The model under review builds one solid part; all positions refer to its coordinate system, in mm. Face numbers are marked on the shaded views. Coordinates: 2 decimals unless noted, no trailing zeros. Order: outer loops, then holes, each group sorted by start corner. A loop starts at its lowest first (then second) coordinate and runs counter-clockwise, first axis right, second up. Notation, with made-up numbers: M -6,50.5 L 10,50.5 A17 cw 10,54.5 Z; hole C 9.25,1.5 d11. An arc over 180 degrees is marked long. Answer as CSV lines item,"result". Start each with the question number.
Q1. For P1, Ø1.3, axis at y = 8.5, z = -5, coming from the +X side; P2, Ø2.5, axis at x = 3, y = -0.5, coming from the -Z side; P3, Ø3, axis at x = 24, y = 9.5, coming from the +Z side; P4, Ø1.3, axis at y = -12, z = 1, coming from the -X side, all flat-tipped, find the tip position at first contact; note any pin that passes through.
Q2. Consider section C-C on x = 32. Write out the cut boundary in (y, z), and give its area (3 significant figures).
Q3. Consider section D-D on x = 18.5. Write out the cut boundary in (y, z), and give its area (3 significant figures).
Q4. Wall thickness on L1, parallel to Z at x = 8.6, y = 0; L2, parallel to Y at x = 10.65, z = 0: over which ranges is each line inside the solid? List them lowest first. Write a range as [from, to].
Q5. The part is to be moulded in two halves that separate along Z. For the marked faces 1, 2 and 3, say which applies: +Z half, -Z half, draft (parallel to the pull), parting line (faces both ways), or undercut.
Q6. Consider section A-A on x = 4. Write out the cut boundary in (y, z), and give its area (3 significant figures).
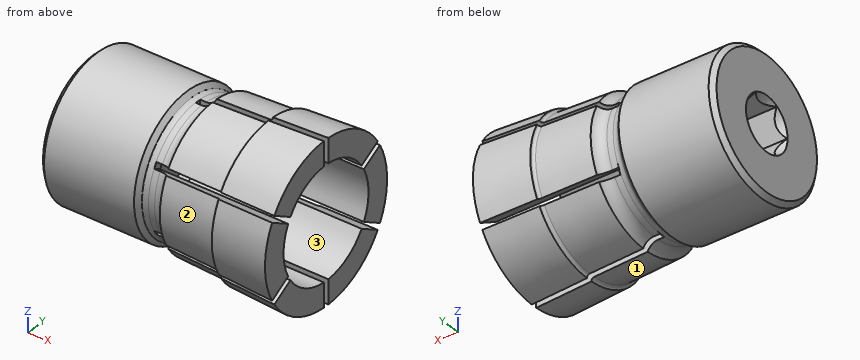
from build123d import *

# Parameters (mm, degrees)
CUT_EXTRUDE1_DEPTH = 6
CUT_EXTRUDE2_DEPTH = 40


with BuildPart() as part:
    # Sketch1 → Revolve1 (revolve)
    with BuildSketch(Plane.XY):
        with BuildLine():
            Line((8.054036255, 0), (0, 4.65))
            Line((0, 4.65), (0, 11.233))
            Line((0, 11.233), (0.767, 12))
            Line((0.767, 12), (16.233, 12))
            Line((16.233, 12), (16.999844549, 11.233155451))
            ThreePointArc((16.999844549, 11.233155451), (17.454138269, 11.059163956), (17.937, 11))
            Line((17.937, 11), (19, 11))
            ThreePointArc((19, 11), (20.115234375, 11.339803539), (20.851508163, 12.243747712))
            Line((20.851508163, 12.243747712), (30.021033995, 12.62983301))
            ThreePointArc((30.021033995, 12.62983301), (30.360913423, 12.783353536), (30.5, 13.129390385))
            Line((30.5, 13.129390385), (30.5, 13.175))
            Line((30.5, 13.175), (40, 13.65))
            Line((40, 13.65), (40, 0))
            Line((40, 0), (8.054036255, 0))
        make_face()
    revolve(axis=Axis((40, 0, 0), (-1, 0, 0)))

    # Sketch2 → Cut-Extrude1 (cut)
    with BuildSketch(Plane(origin=(0, 0, 0), x_dir=(0, 0, -1), z_dir=(1, 0, 0))):
        Polygon((-4, -2.309401077), (0, -4.618802154), (4, -2.309401077), (4, 2.309401077), (0, 4.618802154), (-4, 2.309401077), align=None)
    extrude(amount=CUT_EXTRUDE1_DEPTH, mode=Mode.SUBTRACT)

    # Sketch3 → Cut-Revolve1 (revolve, cut)
    with BuildSketch(Plane(origin=(0, 0, 0), x_dir=(1, 0, 0), z_dir=(0, 1, 0))):
        Polygon((6, 0), (6, 4.75), (8, 4.75), (8, 3.5), (10, 3.5), (10, 9.7), (12, 9.7), (12, 9.5), (42, 9.5), (42, 0), align=None)
    revolve(axis=Axis((42, 0, 0), (-1, 0, 0)), mode=Mode.SUBTRACT)

    # Sketch4 → Cut-Extrude2 (cut)
    with BuildSketch(Plane(origin=(18, 0, 0), x_dir=(0, 0, -1), z_dir=(1, 0, 0))):
        Polygon((-18.65, 0.5), (-18.65, -0.5), (-0.866025404, -0.5), (-9.758012702, -15.901373781), (-8.891987298, -16.401373781), (0, -1), (8.891987298, -16.401373781), (9.758012702, -15.901373781), (0.866025404, -0.5), (18.65, -0.5), (18.65, 0.5), (0.866025404, 0.5), (9.758012702, 15.901373781), (8.891987298, 16.401373781), (0, 1), (-8.891987298, 16.401373781), (-9.758012702, 15.901373781), (-0.866025404, 0.5), align=None)
    extrude(amount=CUT_EXTRUDE2_DEPTH, mode=Mode.SUBTRACT)


solid = part.part
Evaluation:
1,P1,"stops at x = 40"
1,P2,"stops at z = -12"
1,P3,"stops at z = 9.45"
1,P4,"stops at x = 0.16"
2,outline,"M -11.72,-6.19 L -8.47,-4.31 A9.5 cw -8.47,4.31 L -11.72,6.19 A13.25 ccw Z; M -11.22,-7.05 A13.25 ccw -0.5,-13.24 L -0.5,-9.49 A9.5 cw -7.97,-5.18 Z; M -11.22,7.05 L -7.97,5.18 A9.5 cw -0.5,9.49 L -0.5,13.24 A13.25 ccw Z; M 0.5,-13.24 A13.25 ccw 11.22,-7.05 L 7.97,-5.18 A9.5 cw 0.5,-9.49 Z; M 0.5,9.49 A9.5 cw 7.97,5.18 L 11.22,7.05 A13.25 ccw 0.5,13.24 Z; M 8.47,-4.31 L 11.72,-6.19 A13.25 ccw 11.72,6.19 L 8.47,4.31 A9.5 cw Z"
2,area,"246 mm²"
3,outline,"M -9.77,-5.06 L -8.47,-4.31 A9.5 cw -8.47,4.31 L -9.77,5.06 A11 ccw Z; M -9.27,-5.93 A11 ccw -0.5,-10.99 L -0.5,-9.49 A9.5 cw -7.97,-5.18 Z; M -9.27,5.93 L -7.97,5.18 A9.5 cw -0.5,9.49 L -0.5,10.99 A11 ccw Z; M 0.5,-10.99 A11 ccw 9.27,-5.93 L 7.97,-5.18 A9.5 cw 0.5,-9.49 Z; M 0.5,9.49 A9.5 cw 7.97,5.18 L 9.27,5.93 A11 ccw 0.5,10.99 Z; M 8.47,-4.31 L 9.77,-5.06 A11 ccw 9.77,5.06 L 8.47,4.31 A9.5 cw Z"
3,area,"87.6 mm²"
4,L1,"z = [-12, -3.5], [3.5, 12]"
4,L2,"y = [-12, -9.7], [9.7, 12]"
5,face 1,"-Z half"
5,face 2,"parting line"
5,face 3,"undercut"
6,outline,"C 0,0 d24; hole M -4.62,0 L -2.31,-4 L 2.31,-4 L 4.62,0 L 2.31,4 L -2.31,4 Z"
6,area,"397 mm²"
